```python
from build123d import *

# Parameters (mm, degrees)
PAD_DEPTH       = 10
PAD001_DEPTH    = 2.45
POCKET_DEPTH    = 7
SKETCH003_R     = 2.65
POCKET001_DEPTH = 13.751
SKETCH004_R     = 2.65
POCKET002_DEPTH = 5


with BuildPart() as part:
    # Sketch → Pad (new body, symmetric)
    with BuildSketch(Plane.XZ):
        Polygon((0, 14.142136), (-14.142136, 0), (14.142136, 0), (8.803479, 5.338656), (9.86414, 6.399316), (6.399316, 9.86414), (5.338656, 8.803479), align=None)
    extrude(amount=PAD_DEPTH, both=True)

    # Sketch001 → Pad001 (join, symmetric)
    with BuildSketch(Plane.XZ):
        Polygon((0, 14.142136), (-14.142136, 0), (-15.202796, 1.06066), (-1.06066, 15.202796), align=None)
    extrude(amount=PAD001_DEPTH, both=True)

    # Sketch002 → Pocket (cut, symmetric)
    with BuildSketch(Plane.XZ):
        Polygon((-9.899495, 0), (0, 9.899495), (9.899495, 0), align=None)
    extrude(amount=POCKET_DEPTH, both=True, mode=Mode.SUBTRACT)

    # Sketch003 (on Face13 of Pocket) → Pocket001 (cut, through all)
    with BuildSketch(Plane(origin=(4.949747, 0, 4.949747), x_dir=(0.707107, 0, -0.707107), z_dir=(-0.707107, 0, -0.707107))):
        Circle(SKETCH003_R)
    extrude(amount=-POCKET001_DEPTH, mode=Mode.SUBTRACT)

    # Sketch004 (on Face22 of Pocket001) → Pocket002 (cut)
    with BuildSketch(Plane(origin=(-4.949747, 0, 4.949747), x_dir=(0.707107, 0, 0.707107), z_dir=(0.707107, 0, -0.707107))):
        Circle(SKETCH004_R)
    extrude(amount=-POCKET002_DEPTH, mode=Mode.SUBTRACT)


solid = part.part
```
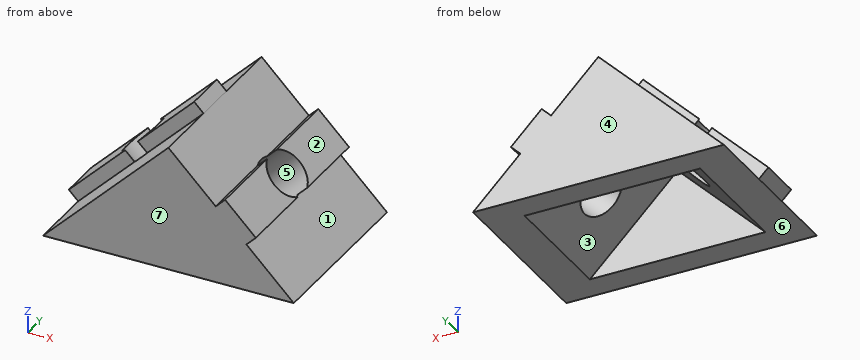
Design review of the part built by this model. Coordinates are the model's own, in mm. Face numbers are marked on the shaded views. A direction names the side the tool comes from. Give positions to 0.01 mm unless a question says otherwise; leave off trailing zeros. Write each loop counter-clockwise with the first axis right and the second up, starting at its lowest first coordinate (ties: lowest second). Pieces come first, ordered by that corner, then holes. Notation, with made-up numbers: (-20.75, 14.5) - (24.25, 14.5) arc R11 cw to (24.25, 34.5) - close; hole circle Ø6 at (75, 38). An arc over 180 degrees is marked (long way). Return JSON: item names as keys, results as strings. Group by question number.
(1) Mouldability with a two-part tool opening along Y and no side actions: class the marked faces 4, 5, 6 and 7 as +Y half, -Y half, draft (parallel to the pull), parting line (faces both ways), or undercut.
(2) We need section B-B, the plane z = 11. Give the boundary of the cut face in (x, y), then the cut area to 3 significant figures.
(3) We need section C-C, the plane x = -2.5. Give the boundary of the cut face in (y, z), then the cut area to 3 significant figures.
(4) Machinability: for the marked faces 1, 2 and 3, which of the approach directions +Z, -Z, +X, -X, +Y, -Y give a long, thin tool a straight path to every point of the face, cutting with its end or side? Answer none if there is none.
(5) We need section D-D, the plane z = 1.5. Give the boundary of the cut face in (x, y).
(6) We need section A-A, the plane y = 7.5. Give the boundary of the cut face in (x, z).
(7) Insertion check: pin 1 (3.5 mm diameter, centred on x = -11.5, z = 3.5, fed in from +Y); pin 2 (12 mm diameter, centred on x = -8.5, y = -6.5, fed in from +Z); pin 3 (10 mm diameter, centred on x = 6.5, y = 5.5, fed in from +Z). Each pin has a flat end and moves straight along its axis. Give the tip position at first contact, or say it passes through.
(8) To check wall thickness, follow probe 1 along Y at (x, z) = (-10.5, 4.75); probe 2 along Y at (x, z) = (1, 6.75); probe 3 along Z at (x, y) = (9, -8.5). State the ranges of each line that lie inside material, in increasing order.
Reported:
{
 "1": {"face 4": "+Y half", "face 5": "undercut", "face 6": "draft", "face 7": "-Y half"},
 "2": {"outline": "(-5.26, -2.45) - (-3.14, -2.45) - (-3.14, -10) - (3.14, -10) - (3.14, 10) - (-3.14, 10) - (-3.14, 2.45) - (-5.26, 2.45) - close", "area": "136 mm2"},
 "3": {"outline": "(-10, 0) - (-7, 0) - (-7, 7.4) - (7, 7.4) - (7, 0) - (10, 0) - (10, 11.64) - (2.45, 11.64) - (2.45, 13.76) - (-2.45, 13.76) - (-2.45, 11.64) - (-10, 11.64) - close", "area": "140 mm2"},
 "4": {"face 1": "+X, +Y, -Y", "face 2": "+Z, +X, +Y, -Y", "face 3": "-Z"},
 "5": {"outline": "(-14.76, -2.45) - (-12.64, -2.45) - (-12.64, -10) - (12.64, -10) - (12.64, 10) - (-12.64, 10) - (-12.64, 2.45) - (-14.76, 2.45) - close; hole (-8.4, -7) - (8.4, -7) - (8.4, 7) - (-8.4, 7) - close"},
 "6": {"outline": "(-14.14, 0) - (14.14, 0) - (8.8, 5.34) - (9.86, 6.4) - (6.4, 9.86) - (5.34, 8.8) - (0, 14.14) - close"},
 "7": {"pin 1": "stops at y = 10", "pin 2": "stops at z = 12.19", "pin 3": "stops at z = 12.64"},
 "8": {"probe 1": "y = -2.45 to 2.45", "probe 2": "y = -10 to -7, 7 to 10", "probe 3": "z = 0 to 5.14, 5.54 to 7.26"}
}
